Check sheet for the modelled part. Datum: model origin and axes. Units: mm. A direction names the side the tool comes from. Give positions to 0.01 mm unless a question says otherwise; leave off trailing zeros. Order: outer loops, then holes, each group sorted by start corner. A loop starts at its lowest first (then second) coordinate and runs counter-clockwise, first axis right, second up. Notation, with made-up numbers: (69.25, 21) -> (100.25, 21) arc R32 ccw to (100.25, 48) -> close; hole circle Ø5 at (-1.5, 19.25). An arc over 180 degrees is marked (long way). One line per question, with ' | ' between items. Start each with the question number.
from build123d import *

# Parameters (mm, degrees)
F0_W     = 570
F0_H     = 290
F1_DEPTH = 230
F3_DEPTH = 40
F4_R     = 19.99999


# Not quite as in the source:
# - a fillet or chamfer is up to 0.001 mm smaller than in the source, because OpenCascade refuses the exact size
# - a feature of the source that left no trace in its solid (it failed there, or was rolled back) is left out


with BuildPart() as f1:
    # F0 (on Top) → F1 (new body)
    with BuildSketch(Plane.XY):
        with Locations((285, -145)):
            Rectangle(F0_W, F0_H)
    extrude(amount=F1_DEPTH)

    # F2 (on face) → F3 (cut)
    with BuildSketch(Plane.XY.offset(230)):
        Polygon((0, -220), (250, -220), (250, -145), (250, -70), (0, -70), (0, -145), align=None)
    extrude(amount=-F3_DEPTH, mode=Mode.SUBTRACT)

    # F4 (radius 20 in the source; OpenCascade refuses exactly that, so slightly less here)
    f4_edges = [f1.edges().sort_by_distance(p)[0] for p in [
        (0, -145, 0),
        (0, -290, 115),
        (0, -255, 230),
        (0, -220, 210),
        (0, -145, 190),
        (0, -70, 210),
        (0, -35, 230),
        (0, 0, 115),
        (570, -290, 115),
        (570, 0, 115),
        (570, -145, 0),
        (570, -145, 230),
        (285, -290, 0),
        (285, -290, 230),
        (285, 0, 0),
        (285, 0, 230),
        (125, -220, 190),
        (250, -145, 190),
        (125, -70, 190),
        (125, -220, 230),
        (250, -145, 230),
        (125, -70, 230),
    ]]
    fillet(f4_edges, radius=F4_R)


solid = f1.part
1. Mould release check, pull along Y, two halves, no side actions. Record for faces 3 (the face through (133.39, -75.703, 196.014)), 4 (the face through (288.71, -283.986, 5.703)), 5 (the face through (288.71, -6.014, 5.703)): +Y half, -Y half, draft (parallel to the pull), parting line (faces both ways), or undercut.
2. Go/stop test with a flat-tipped pin: pin 1 (12 mm diameter, centred on x = 173, y = -122, fed in from +Z). Record where the tip stops, or that it passes through.
3. Scan lines: probe 1 along X at (y, z) = (-78, 173); probe 2 along Z at (x, y) = (114, -53); probe 3 along Z at (x, y) = (231, -92.5). Record each from-to range of solid material in increasing order.
4. Cross-section at C-C on x = 257. Record the boundary of the cut face in (y, z).
5. Tool access check on faces 1 (the face through (136.61, -213.986, 195.703)), 2 (the face through (5.703, -6.014, 116.33)). Record the directions out of +Z, -Z, +X, -X, +Y, -Y that give a thin tool (end or side, any length) a straight path to the whole face; none if there is none.
Response values:
1) face 3: undercut | face 4: -Y half | face 5: +Y half
2) pin 1: stops at z = 190
3) probe 1: x = 0.03 to 570 | probe 2: z = 0 to 229.77 | probe 3: z = 0 to 190.03
4) outline: (-290, 20) arc R20 ccw to (-270, 0) -> (-20, 0) arc R20 ccw to (0, 20) -> (0, 210) arc R20 ccw to (-20, 230) -> (-50, 230) arc R20 ccw to (-63, 225.2) -> (-227, 225.2) arc R20 ccw to (-240, 230) -> (-270, 230) arc R20 ccw to (-290, 210) -> close
5) face 1: +Z, -X | face 2: +Z, -Z, -X, +Y
